Autodesk Inventor part; units mm, degrees
ref_plane "Work Plane1" through (-9, 33.5885, 16.5511) normal (1, 0, 0) x (0, 0, -1)
ref_plane "YZ Plane" through (0, 0, 0) normal (1, 0, 0) x (0, 1, 0)
ref_plane "XZ Plane" through (0, 0, 0) normal (0, 1, 0) x (-1, 0, 0)
sketch "Sketch1" plane through (0, 0, 0) normal (0, 1, 0) x (-1, 0, 0)
  line L0 (0, 0) -> (18, 0)
  line L1 (18, 0) -> (18, 18)
  line L2 (18, 18) -> (0, 18)
  line L3 (0, 18) -> (0, 0)
  dimension "d0" = 18
  dimension "d1" = 18
extrude "Extrusion1" add sketch "Sketch1" along normal blind 8 draft -15
fillet "Fillet1" radius 1.5 8 edges at (-1.0718, 4, 16.9282) (-9, 8, 15.8564) (-2.1436, 8, 9) (-9, 8, 2.1436) (-1.0718, 4, 1.0718) (-16.9282, 4, 1.0718) (-16.9282, 4, 16.9282) (-15.8564, 8, 9)
ref_plane "Work Plane1" through (-9, 33.5885, 16.5511) normal (1, 0, 0) x (0, 0, -1)
sketch "Sketch2" plane through (-9, 33.5885, 16.5511) normal (1, 0, 0) x (0, 0, -1)
  line L0 (13.2565, -25.5885) -> (1.8457, -25.5885)
  arc A0 (14.7054, -26.7002) -> (13.2565, -25.5885) centre (13.2565, -27.0885) ccw
  arc A1 (1.8457, -25.5885) -> (13.2565, -25.5885) centre (7.5511, -8.5166) ccw
  point P0 (16.5511, -33.5885)
  point P1 (13.2565, -25.5885)
  dimension "d5" = 18
extrude "Extrusion2" cut sketch "Sketch2" along normal through all both and the other way through all
sketch "Sketch3" plane through (0, 0, 0) normal (0, -1, 0) x (1, 0, 0)
  line L0 (-16.5511, 18) -> (-1.4489, 18) construction
  line L1 (-9, 18) -> (-9, 0) construction
  line L2 (-1.4489, 0) -> (-16.5511, 0) construction
  line L3 (-18, 1.4489) -> (-18, 16.5511) construction
  line L4 (-18, 9) -> (0, 9) construction
  line L5 (-1, 1) -> (-17, 1)
  line L6 (-17, 1) -> (-17, 17)
  line L7 (-17, 17) -> (-1, 17)
  line L8 (-1, 17) -> (-1, 1)
  line L9 (-1, 1) -> (-17, 17) construction
  line L10 (-17, 1) -> (-1, 17) construction
  point P0 (0, 0)
  point P1 (-9, 9)
  point P2 (-9, 9)
  dimension "d8" = 16
  dimension "d9" = 16
extrude "Extrusion3" cut sketch "Sketch3" against normal blind 4.5 draft -15
sketch "Sketch4" plane through (0, 4.5, 0) normal (0, -1, 0) x (1, 0, 0)
  line L0 (-15.7942, 15.7942) -> (-15.7942, 2.2058) construction
  line L1 (-15.7942, 9) -> (-2.2058, 9) construction
  line L2 (-2.2058, 2.2058) -> (-2.2058, 15.7942) construction
  line L3 (-2.2058, 15.7942) -> (-15.7942, 15.7942) construction
  line L4 (-9, 15.7942) -> (-9, 2.2058) construction
  line L5 (-15.7942, 2.2058) -> (-2.2058, 2.2058) construction
  circle A0 centre (-9, 9) radius 2.775
  point P0 (0, 0)
  dimension "d12" = 5.55
extrude "Extrusion4" add sketch "Sketch4" along normal blind 4
sketch "Sketch5" plane through (-9, 0.5, 9) normal (0, -1, 0) x (1, 0, 0)
  line L0 (0.6, 2.075) -> (-0.6, 2.075)
  line L1 (-0.6, -2.075) -> (0.6, -2.075)
  line L2 (-0.6, 2.075) -> (0.6, -2.075) construction
  line L3 (-2.075, 0.6) -> (-2.075, -0.6)
  line L4 (2.075, -0.6) -> (2.075, 0.6)
  line L5 (2.075, 0.6) -> (-2.075, -0.6) construction
  line L6 (-2.075, 0.6) -> (2.075, -0.6) construction
  line L7 (-6.7942, 6.7942) -> (-6.7942, -6.7942) construction
  line L8 (-6.7942, 0) -> (6.7942, 0) construction
  line L9 (6.7942, -6.7942) -> (6.7942, 6.7942) construction
  line L10 (-6.7942, -6.7942) -> (6.7942, -6.7942) construction
  line L11 (0, -6.7942) -> (0, 6.7942) construction
  arc A0 (0.9, -0.6) -> (0.6, -0.9) centre (0.9, -0.9) ccw
  arc A1 (-0.6, -0.9) -> (-0.9, -0.6) centre (-0.9, -0.9) ccw
  arc A2 (0.6, 0.9) -> (0.9, 0.6) centre (0.9, 0.9) ccw
  arc A3 (-0.9, 0.6) -> (-0.6, 0.9) centre (-0.9, 0.9) ccw
  line L12 (-0.6, 2.075) -> (-0.6, 0.9)
  line L13 (-0.6, -0.9) -> (-0.6, -2.075)
  line L14 (-2.075, -0.6) -> (-0.9, -0.6)
  line L15 (-0.9, 0.6) -> (-2.075, 0.6)
  line L16 (0.6, 2.075) -> (0.1735, 0.6) construction
  line L17 (0, 0) -> (-0.6, -2.075) construction
  line L18 (2.075, 0.6) -> (0.9, 0.6)
  line L19 (0.9, -0.6) -> (2.075, -0.6)
  line L20 (0.6, -2.075) -> (0.6, -0.9)
  line L21 (0.6, 0.9) -> (0.6, 2.075)
  point P0 (9, -9)
  dimension "d15" = 1.2
  dimension "d16" = 4.15
  dimension "d17" = 4.15
  dimension "d18" = 1.2
  dimension "d19" = 0.3
extrude "Extrusion5" cut sketch "Sketch5" against normal blind 4
ref_plane "Work Plane3" through (0, 6, 0) normal (0, -1, 0) x (1, 0, 0)
split_face "Split1"
sketch "Sketch7" plane through (0, 6, 0) normal (0, -1, 0) x (1, 0, 0)
  line L0 (-25.6931, 27.6788) -> (12.1363, 27.6788)
  line L1 (12.1363, 27.6788) -> (12.1363, -37.3947)
  line L2 (12.1363, -37.3947) -> (-25.6931, -37.3947)
  line L3 (-25.6931, -37.3947) -> (-25.6931, 27.6788)
  point P0 (0, 0)
extrude "Extrusion7" cut sketch "Sketch7" along normal blind 10
properties part number "top"
Source: CAD feature listing. Evaluate the final solid. Frame: model axes, mm. Coordinates: 2 decimals unless noted, no trailing zeros. Loops run counter-clockwise (first coordinate to the right, second up) from the corner with the lowest first, then second, coordinate; pieces in that order, holes last. Notation, with made-up numbers: (56.5, 0.5) - (78.5, 0.5) arc R21 cw to (78.5, 25.5) - close; hole circle Ø6 at (40, 9). An arc over 180 degrees is marked (long way). Return JSON: item names as keys, results as strings.
Q1. Section A-A, the plane y = 7.35. Return loops of the section in (x, z).
Results:
{"outline": "(-15.94, 3.29) arc R1.24 ccw to (-14.71, 2.06) - (-3.29, 2.06) arc R1.24 ccw to (-2.06, 3.29) - (-2.06, 5.85) - (-15.94, 5.85) - close; (-15.94, 12.15) - (-2.06, 12.15) - (-2.06, 14.71) arc R1.24 ccw to (-3.29, 15.94) - (-14.71, 15.94) arc R1.24 ccw to (-15.94, 14.71) - close"}
Q2. Material intervals for line 1 along X through (y, z) = (6.9, 5.5); line 2 along Z through (x, y) = (-12.25, 6.2); line 3 along Y through (x, z) = (-2.5, 4), sorted ascending.
Results:
{"line 1": "-16.15 to -1.85", "line 2": "1.66 to 16.34", "line 3": "6 to 7.77"}
Q3. Section D-D, the plane z = 11.75. Return loops of the section in (x, y).
Results:
{"outline": "(-16.39, 6) - (-1.61, 6) - (-1.85, 6.89) arc R1.5 ccw to (-2.02, 7.28) - (-15.98, 7.28) arc R1.5 ccw to (-16.15, 6.89) - close"}
Q4. Mould query, pull axis Z, two halves, no side actions, for faces 1 (the flat face through (-1.725, 6.438, 8.917)), 2 (the flat face through (-8.917, 6.438, 16.275)), 3 (the cylindrical face through (-2.155, 6.523, 2.178)), 4 (the cylindrical face through (-9.099, 7.072, 8.919)). Classes: released by +Z, released by -Z, zero draft, split by the parting line, or undercut.
Results:
{"face 1": "zero draft", "face 2": "released by +Z", "face 3": "released by -Z", "face 4": "undercut"}
Q5. Section C-C, the plane z = 9. Return loops of the section in (x, y), plus the area to 3 significant figures.
Results:
{"outline": "(-16.39, 6) - (-1.61, 6) - (-1.85, 6.89) arc R1.5 ccw to (-1.91, 7.07) - (-16.09, 7.07) arc R1.5 ccw to (-16.15, 6.89) - close", "area": "15.5 mm2"}
